The figure shows three views and two pictorial views of one solid part (mm, origin at its lowest corner). Answer the questions. A direction names the side the tool comes from. Round coordinates to 2 decimals unless told otherwise and drop trailing zeros. Order: outer loops, then holes, each group sorted by start corner. A loop starts at its lowest first (then second) coordinate and runs counter-clockwise, first axis right, second up. Notation, with made-up numbers: M 18.25,16.25 L 74.25,16.25 A18 cw 74.25,23.25 Z; hole C 54,-16 d4. An arc over 180 degrees is marked long. Return JSON: item names as keys, results as strings.
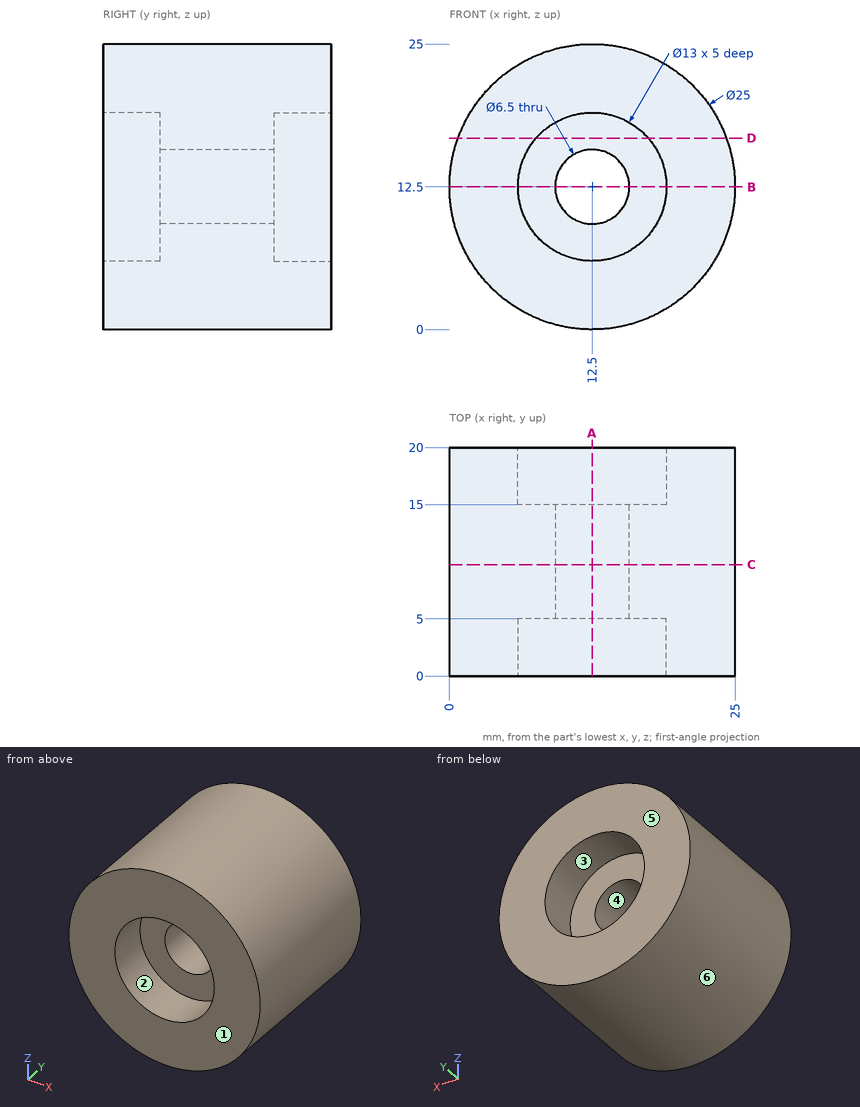
Item 1: Find section C-C (y = 9.75). Determine the outline of the cut face in (x, z), plus the area to 3 significant figures.
Output:
{"outline": "C 12.5,12.5 d25; hole C 12.5,12.5 d6.5", "area": "458 mm^2"}
Item 2: The mould has two halves that part along X. Classify the marked faces 4, 5 and 6: pulls with the +X half, pulls with the -X half, needs draft (parallel to the pull), parting line crosses it, or undercut.
Output:
{"face 4": "undercut", "face 5": "needs draft", "face 6": "parting line crosses it"}
Item 3: Find section A-A (x = 12.5). Determine the outline of the cut face in (y, z), plus the area to 3 significant figures.
Output:
{"outline": "M 0,0 L 20,0 L 20,6 L 15,6 L 15,9.25 L 5,9.25 L 5,6 L 0,6 Z; M 0,19 L 5,19 L 5,15.75 L 15,15.75 L 15,19 L 20,19 L 20,25 L 0,25 Z", "area": "305 mm^2"}
Item 4: Which of the six approach directions +Z, -Z, +X, -X, +Y, -Y give full straight-line access (tool end or side, diameter ignored) to the marked faces 1, 2 and 3?
Output:
{"face 1": "+Z, -Z, +X, -X, -Y", "face 2": "-Y", "face 3": "+Y"}
Item 5: Consider line 1 along Z through (x, y) = (12.5, 1.75); line 2 along Z through (x, y) = (12.5, 9.75). Determine where each line is inside the solid, lowest interval first. Write a range as [from, to].
Output:
{"line 1": "z = [0, 6], [19, 25]", "line 2": "z = [0, 9.25], [15.75, 25]"}
Item 6: Find section D-D (z = 16.75). Determine the outline of the cut face in (x, y), plus the area to 3 significant figures.
Output:
{"outline": "M 0.74,0 L 7.58,0 L 7.58,5 L 17.42,5 L 17.42,0 L 24.26,0 L 24.26,20 L 17.42,20 L 17.42,15 L 7.58,15 L 7.58,20 L 0.74,20 Z", "area": "372 mm^2"}
Item 7: Find section B-B (z = 12.5). Determine the outline of the cut face in (x, y), plus the area to 3 significant figures.
Output:
{"outline": "M 0,0 L 6,0 L 6,5 L 9.25,5 L 9.25,15 L 6,15 L 6,20 L 0,20 Z; M 15.75,5 L 19,5 L 19,0 L 25,0 L 25,20 L 19,20 L 19,15 L 15.75,15 Z", "area": "305 mm^2"}
Item 8: Each of these flat-tipped pins is pushed along its axis until it touches: pin 1 (3 mm diameter, centred on y = 5, z = 8, fed in from +X); pin 2 (10 mm diameter, centred on x = 4, y = 16.5, fed in from -Z); pin 3 (10.5 mm diameter, centred on x = 12.5, z = 12.5, fed in from +Y). Where does it stop, or does it pass through?
Output:
{"pin 1": "stops at x = 24.63", "pin 2": "stops at z = 0.5", "pin 3": "stops at y = 15"}
